Verification items for the finished model (mm, model axes). Face numbers are marked on the shaded views. A direction names the side the tool comes from. Round coordinates to 2 decimals unless told otherwise and drop trailing zeros. Order: outer loops, then holes, each group sorted by start corner. A loop starts at its lowest first (then second) coordinate and runs counter-clockwise, first axis right, second up. Notation, with made-up numbers: M 45,24 L 89,24 A15 cw 89,39 Z; hole C 85,38 d9. An arc over 180 degrees is marked long. Use one line per item in the form item = value. Start each with the question number.
Item 1: Release check for a two-part mould opening along Z. For the marked faces 1, 2, 3 and 4 record: +Z half, -Z half, draft (parallel to the pull), parting line (faces both ways), or undercut.
Item 2: Tool access check on the marked faces 5, 6 and 7. Record the directions out of +Z, -Z, +X, -X, +Y, -Y that give a thin tool (end or side, any length) a straight path to the whole face; none if there is none.
Item 3: Thickness scan on probe 1 along X at (y, z) = (-5, 24.5); probe 2 along Z at (x, y) = (11, -1); probe 3 along Z at (x, y) = (-7.5, -10.25). Record the ranges inside material, lowest first. Write a range as [from, to].
Item 4: Go/stop test with flat-tipped pins: pin 1 Ø1.9 at (x, z) = (8, 28) entering from +Y; pin 2 Ø2 at (x, z) = (-15.09, 19.69) entering from +Y; pin 3 Ø6 at (x, z) = (-25, 25.5) entering from -Y; pin 4 Ø1.5 at (x, z) = (3.5, 22.5) entering from -Y. Record where each tip stops, or that it passes through.
Item 5: Cross-section at B-B on z = 23.5. Enter the section's corners in (x, y).
Item 6: Cross-section at C-C on x = -18.5. Enter the section's corners in (y, z).
Item 7: Cross-section at A-A on y = -10.25. Count the separate pieces of the cut face and the enclosed holes in it, then the cut area to 3 significant figures.
Item 8: Cross-section at D-D on y = -6.5. Enter the section's corners in (x, z), then the cut area to 3 significant figures.
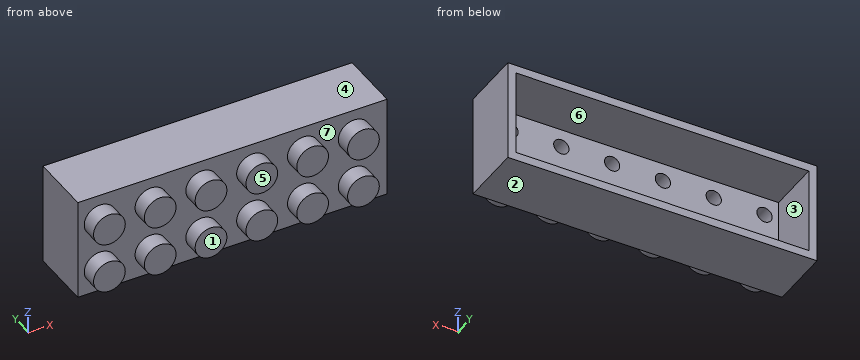
from build123d import *

# Parameters (mm, degrees)
F0_W     = 47.752
F0_H     = 15.7988
F1_DEPTH = 9.53
F2_R     = 2.4511
F3_DEPTH = 2.54
F4_T     = -1.27


with BuildPart() as f1:
    # F0 (on Front) → F1 (new body)
    with BuildSketch(Plane.XZ):
        with Locations((-10.3473756462, 23.7146833966)):
            Rectangle(F0_W, F0_H)
    extrude(amount=F1_DEPTH)

    # F2 (on face) → F3 (join)
    with BuildSketch(Plane.XZ.offset(9.53)):
        with Locations((8.4527879953, 27.5373833966)):
            Circle(F2_R)
        with Locations((8.4527879953, 19.6887833966)):
            Circle(F2_R)
        with Locations((0.6041879953, 27.5373833966)):
            Circle(F2_R)
        with Locations((0.6041879953, 19.6887833966)):
            Circle(F2_R)
        with Locations((-7.2444120047, 27.5373833966)):
            Circle(F2_R)
        with Locations((-7.2444120047, 19.6887833966)):
            Circle(F2_R)
        with Locations((-15.0930120047, 27.5373833966)):
            Circle(F2_R)
        with Locations((-15.0930120047, 19.6887833966)):
            Circle(F2_R)
        with Locations((-22.9416120047, 27.5373833966)):
            Circle(F2_R)
        with Locations((-22.9416120047, 19.6887833966)):
            Circle(F2_R)
        with Locations((-30.7902120047, 27.5373833966)):
            Circle(F2_R)
        with Locations((-30.7902120047, 19.6887833966)):
            Circle(F2_R)
    extrude(amount=F3_DEPTH)

    # F4
    f4_openings = [f1.faces().sort_by_distance(p)[0] for p in [
        (-10.347376, 0, 23.714683),
    ]]
    offset(amount=F4_T, openings=f4_openings, kind=Kind.INTERSECTION)


solid = f1.part
Output values:
q1.face_1 = draft
q1.face_2 = -Z half
q1.face_3 = undercut
q1.face_4 = +Z half
q2.face_5 = +Z, -Z, +X, -X, -Y
q2.face_6 = +Y
q2.face_7 = -Y
q3.probe_1 = [-34.22, -32.95], [12.26, 13.53]
q3.probe_2 = [15.82, 17.09], [30.34, 31.61]
q3.probe_3 = [17.25, 18.54], [20.84, 22.13], [25.1, 26.38], [28.69, 29.98]
q4.pin_1 = -8.26
q4.pin_2 = -10.8
q4.pin_3 = -12.07
q4.pin_4 = -9.53
q5.outline = M -34.22,-9.53 L 13.53,-9.53 L 13.53,0 L 12.26,0 L 12.26,-8.26 L -32.95,-8.26 L -32.95,0 L -34.22,0 Z
q6.outline = M -9.53,15.82 L 0,15.82 L 0,17.09 L -8.26,17.09 L -8.26,30.34 L 0,30.34 L 0,31.61 L -9.53,31.61 Z
q7.separate_pieces = 12
q7.enclosed_holes = 12
q7.area = 174 mm2
q8.outline = M -34.22,15.82 L 13.53,15.82 L 13.53,31.61 L -34.22,31.61 Z; hole M -32.95,17.09 L 12.26,17.09 L 12.26,30.34 L -32.95,30.34 Z
q8.area = 155 mm2
